Check sheet for the modelled part. Datum: model origin and axes. Units: mm. A direction names the side the tool comes from. Coordinates: 2 decimals unless noted, no trailing zeros. Write each loop counter-clockwise with the first axis right and the second up, starting at its lowest first coordinate (ties: lowest second). Pieces come first, ordered by that corner, then holes. Notation, with made-up numbers: (49, 21) -> (70, 21) arc R19 ccw to (70, 55) -> close; hole circle Ø2 at (-34, 76.25). An arc over 180 degrees is marked (long way). One line per item, written item: value. Start each with the question number.
1) Scan lines: line 1 along X through (y, z) = (35, 6.25) (3 decimals); line 2 along X through (y, z) = (34.5, 0.75) (3 decimals). Record each from-to range of solid material in increasing order. Write a range as [from, to].
2) Draft check along X on faces 3 (the cylindrical face through (0.349, -44.446, 3.131)), 4 (the flat face through (40, 3, 0)). Enter one of: +X half, -X half, draft (parallel to the pull), parting line (faces both ways), or undercut.
3) Sectioned sample at A-A on x = 0. Enter the section's corners in (y, z), plus the area to 3 significant figures.
4) Set-up check for faces 1 (the flat face through (40, 3, 6.35)), 2 (the cylindrical face through (-0.349, 44.446, 3.131)): record each of +Z, -Z, +X, -X, +Y, -Y from which the full face is reachable in a straight line by a thin tool's end or side.
```python
from build123d import *

# Parameters (mm, degrees)
F0_W     = 387.35
F0_H     = 479.425
F1_DEPTH = 6.35


with BuildPart() as f1:
    # F0 (on Top) → F1 (new body)
    with BuildSketch(Plane.XY):
        Rectangle(F0_W, F0_H)
        with BuildLine():
            Line((-15.875, -28.575), (-15.875, 28.575))
            ThreePointArc((-15.875, 28.575), (0, 44.45), (15.875, 28.575))
            Line((15.875, 28.575), (15.875, -28.575))
            ThreePointArc((15.875, -28.575), (0, -44.45), (-15.875, -28.575))
        make_face(mode=Mode.SUBTRACT)
    extrude(amount=F1_DEPTH)


solid = f1.part
```
Answers:
1. line 1: x = [-193.675, -14.517], [14.517, 193.675]
1. line 2: x = [-193.675, -14.728], [14.728, 193.675]
2. face 3: undercut
2. face 4: draft
3. outline: (-239.71, 0) -> (-44.45, 0) -> (-44.45, 6.35) -> (-239.71, 6.35) -> close; (44.45, 0) -> (239.71, 0) -> (239.71, 6.35) -> (44.45, 6.35) -> close
3. area: 2,480 mm2
4. face 1: +Z, +X, -X, +Y, -Y
4. face 2: +Z, -Z
